```python
from build123d import *

# Parameters (mm, degrees)
F1_DEPTH = 25.4
F2_T     = -5.08


with BuildPart() as f1:
    # F0 (on Right) → F1 (new body)
    with BuildSketch(Plane.YZ):
        Polygon((-76.2, -25.698823), (0, -25.698823), (0, 75.901177), align=None)
    extrude(amount=F1_DEPTH)

    # F2
    f2_openings = [f1.faces().sort_by_distance(p)[0] for p in [
        (12.7, -38.1, 25.101177),
    ]]
    offset(amount=F2_T, openings=f2_openings)


solid = f1.part
```
Build history of the part. All positions in model axes, mm. A direction names the side the tool comes from. Round coordinates to 2 decimals unless told otherwise and drop trailing zeros. Loops run counter-clockwise (first coordinate to the right, second up) from the corner with the lowest first, then second, coordinate; pieces in that order, holes last. Notation, with made-up numbers: M 7,-5 L 21,-5 A15 ccw 21,4 Z; hole C 28,30 d5. An arc over 180 degrees is marked long. Answer as CSV lines item,"result".
1. Cut at C-C on x = 16.5. Write the cut outline in (y, z), then the cut area to 3 significant figures.
Resolved:
outline,"M -76.2,-25.7 L 0,-25.7 L 0,75.9 L -5.08,69.13 L -5.08,-20.62 L -72.39,-20.62 Z"
area,"851 mm²"
2. Flat gauge pins, fed straight in: P1, Ø4.5, axis at x = 12.5, z = 17, coming from the -Y side; P2, Ø2, axis at x = 20, y = -59, coming from the +Z side; P3, Ø4.5, axis at x = 12, y = -55, coming from the +Z side. Where does each tip first touch, or does it go through?
Resolved:
P1,"stops at y = -5.08"
P2,"stops at z = -1.5"
P3,"stops at z = -20.62"
3. Cut at A-A on z = -2.5. Write the cut outline in (x, y), then the cut area to 3 significant figures.
Resolved:
outline,"M 0,-58.8 L 5.08,-58.8 L 5.08,-5.08 L 20.32,-5.08 L 20.32,-58.8 L 25.4,-58.8 L 25.4,0 L 0,0 Z"
area,"675 mm²"
4. Two-plate mould, pull along X, no slides. Class faces 1 (the flat face through (25.4, -22, 3)), 2 (the flat face through (0, -22, 3)), 3 (the flat face through (13, -5.08, 24)): released by +X, released by -X, zero draft, split by the parting line, or undercut.
Resolved:
face 1,"released by +X"
face 2,"released by -X"
face 3,"undercut"
5. Cut at B-B on y = -62. Write the cut outline in (x, z).
Resolved:
outline,"M 0,-25.7 L 25.4,-25.7 L 25.4,-6.77 L 20.32,-6.77 L 20.32,-20.62 L 5.08,-20.62 L 5.08,-6.77 L 0,-6.77 Z"
6. 3-axis set-ups, long thin cutter, end or side, ignore diameter. For faces 4 (the flat face through (13, -39, -20.619)), 5 (the flat face through (13, -39, -25.699)): which of +Z, -Z, +X, -X, +Y, -Y reach the whole face in a straight line?
Resolved:
face 4,"+Z, -Y"
face 5,"-Z, +X, -X, +Y, -Y"
7. Wall check: probe 1 along X at (y, z) = (-46, 1); probe 2 along Z at (x, y) = (13, -32); probe 3 along Y at (x, z) = (13.25, 18). Give the ranges that are in metal, low to high. Write a range as [from, to].
Resolved:
probe 1,"x = [0, 5.08], [20.32, 25.4]"
probe 2,"z = [-25.7, -20.62]"
probe 3,"y = [-5.08, 0]"
8. Cut at D-D on x = 23.5. Write the cut outline in (y, z), then the cut area to 3 significant figures.
Resolved:
outline,"M -76.2,-25.7 L 0,-25.7 L 0,75.9 Z"
area,"3,870 mm²"
